```python
from build123d import *

# Parameters (mm, degrees)
F0_W     = 38.1
F0_H     = 38.1
F0_H_2   = 368.3
F0_H_3   = 25.4
F1_DEPTH = 38.1
F2_DEPTH = 800.1
F0_W_2   = 768.35
F3_DEPTH = 38.1


with BuildPart() as f1:
    # F0 (on Top) → F1 (new body)
    with BuildSketch(Plane.XY):
        with Locations((1200.15, 590.55)):
            Rectangle(F0_W, F0_H)
        Polygon((1181.1, 571.5), (1181.1, 609.6), (19.05, 609.6), (19.05, 571.5), (374.65, 571.5), (412.75, 571.5), align=None)
        Polygon((1219.2, -571.5), (1219.2, 571.5), (1181.1, 571.5), (1181.1, 203.2), (1181.1, 177.8), (1181.1, 0), (1181.1, -177.8), (1181.1, -203.2), (1181.1, -571.5), align=None)
        Polygon((19.05, 571.5), (19.05, 609.6), (-19.05, 609.6), (-19.05, 571.5), (0, 571.5), align=None)
        with Locations((1200.15, -590.55)):
            Rectangle(F0_W, F0_H)
        Polygon((-19.05, 571.5), (-19.05, 609.6), (-1181.1, 609.6), (-1181.1, 571.5), (-412.75, 571.5), (-374.65, 571.5), align=None)
        Polygon((1181.1, -609.6), (1181.1, -571.5), (412.75, -571.5), (374.65, -571.5), (19.05, -571.5), (19.05, -609.6), align=None)
        with Locations((-1200.15, 590.55)):
            Rectangle(F0_W, F0_H)
        Polygon((-1181.1, 203.2), (-1181.1, 571.5), (-1219.2, 571.5), (-1219.2, -571.5), (-1181.1, -571.5), (-1181.1, -203.2), (-1181.1, -177.8), (-1181.1, 0), (-1181.1, 177.8), align=None)
        with Locations((0, -590.55)):
            Rectangle(F0_W, F0_H)
        Polygon((-1181.1, -609.6), (-19.05, -609.6), (-19.05, -571.5), (-374.65, -571.5), (-412.75, -571.5), (-1181.1, -571.5), align=None)
        with Locations((-1200.15, -590.55)):
            Rectangle(F0_W, F0_H)
        with Locations((-393.7, 387.35)):
            Rectangle(F0_W, F0_H_2)
        with Locations((-393.7, -387.35)):
            Rectangle(F0_W, F0_H_2)
        with Locations((393.7, 387.35)):
            Rectangle(F0_W, F0_H_2)
        with Locations((393.7, -387.35)):
            Rectangle(F0_W, F0_H_2)
        Polygon((412.75, -177.8), (412.75, 0), (393.7, 0), (374.65, 0), (374.65, -177.8), align=None)
        Polygon((412.75, 0), (412.75, 177.8), (374.65, 177.8), (374.65, 0), (393.7, 0), align=None)
        with Locations((393.7, -190.5)):
            Rectangle(F0_W, F0_H_3)
        with Locations((393.7, 190.5)):
            Rectangle(F0_W, F0_H_3)
        with Locations((-393.7, -190.5)):
            Rectangle(F0_W, F0_H_3)
        Polygon((-374.65, -177.8), (-374.65, 0), (-393.7, 0), (-412.75, 0), (-412.75, -177.8), align=None)
        Polygon((-374.65, 0), (-374.65, 177.8), (-412.75, 177.8), (-412.75, 0), (-393.7, 0), align=None)
        with Locations((-393.7, 190.5)):
            Rectangle(F0_W, F0_H_3)
    extrude(amount=F1_DEPTH)

    # F0 (on Top) → F2 (join)
    with BuildSketch(Plane.XY):
        with Locations((1200.15, 590.55)):
            Rectangle(F0_W, F0_H)
        with Locations((1200.15, -590.55)):
            Rectangle(F0_W, F0_H)
        with Locations((0, -590.55)):
            Rectangle(F0_W, F0_H)
        Polygon((19.05, 571.5), (19.05, 609.6), (-19.05, 609.6), (-19.05, 571.5), (0, 571.5), align=None)
        with Locations((-1200.15, 590.55)):
            Rectangle(F0_W, F0_H)
        with Locations((-1200.15, -590.55)):
            Rectangle(F0_W, F0_H)
    extrude(amount=-F2_DEPTH)

    # F0 (on Top) → F3 (join)
    with BuildSketch(Plane.XY):
        Polygon((-374.65, -203.2), (374.65, -203.2), (374.65, -177.8), (0, -177.8), (-374.65, -177.8), align=None)
        Polygon((374.65, 177.8), (374.65, 203.2), (0, 203.2), (0, 190.5), (0, 177.8), align=None)
        with Locations((-796.925, 190.5)):
            Rectangle(F0_W_2, F0_H_3)
        Polygon((0, 190.5), (0, 203.2), (-374.65, 203.2), (-374.65, 177.8), (0, 177.8), align=None)
        with Locations((-796.925, -190.5)):
            Rectangle(F0_W_2, F0_H_3)
        with Locations((796.925, -190.5)):
            Rectangle(F0_W_2, F0_H_3)
        with Locations((796.925, 190.5)):
            Rectangle(F0_W_2, F0_H_3)
    extrude(amount=F3_DEPTH)


solid = f1.part
```
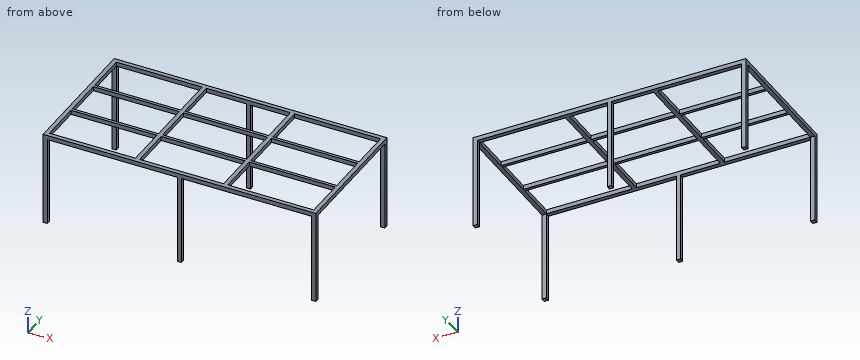
Check sheet for the modelled part. Datum: model origin and axes. Units: mm. Round coordinates to 2 decimals unless told otherwise and drop trailing zeros. Order: outer loops, then holes, each group sorted by start corner. A loop starts at its lowest first (then second) coordinate and runs counter-clockwise, first axis right, second up. Notation, with made-up numbers: (25.5, 19.25) -> (57.5, 19.25) arc R15 cw to (57.5, 30.25) -> close; hole circle Ø9 at (40.25, -9). An arc over 180 degrees is marked (long way). One line per item, written item: value. Start each with the question number.
Q1. Cross-section at A-A (z = -391.5). Record the boundary of the cut face in (x, y), and give its area (3 significant figures).
Q2. Gauge pin test, flat end, axial feed: pin 1 Ø5 at (x, z) = (-22, -183.5) entering from -Y. Record the tip position at first contact, or that the pin passes through.
Q3. Cross-section at B-B (y = -491.5). Record the boundary of the cut face in (x, z).
Q4. Cross-section at C-C (x = -724.5). Record the boundary of the cut face in (y, z), and give its area (3 significant figures).
Completed:
1. outline: (-1219.2, -609.6) -> (-1181.1, -609.6) -> (-1181.1, -571.5) -> (-1219.2, -571.5) -> close; (-1219.2, 571.5) -> (-1181.1, 571.5) -> (-1181.1, 609.6) -> (-1219.2, 609.6) -> close; (-19.05, -609.6) -> (19.05, -609.6) -> (19.05, -571.5) -> (-19.05, -571.5) -> close; (-19.05, 571.5) -> (19.05, 571.5) -> (19.05, 609.6) -> (-19.05, 609.6) -> close; (1181.1, -609.6) -> (1219.2, -609.6) -> (1219.2, -571.5) -> (1181.1, -571.5) -> close; (1181.1, 571.5) -> (1219.2, 571.5) -> (1219.2, 609.6) -> (1181.1, 609.6) -> close
1. area: 8,710 mm²
2. pin 1: passes through
3. outline: (-1219.2, 0) -> (-1181.1, 0) -> (-1181.1, 38.1) -> (-1219.2, 38.1) -> close; (-412.75, 0) -> (-374.65, 0) -> (-374.65, 38.1) -> (-412.75, 38.1) -> close; (374.65, 0) -> (412.75, 0) -> (412.75, 38.1) -> (374.65, 38.1) -> close; (1181.1, 0) -> (1219.2, 0) -> (1219.2, 38.1) -> (1181.1, 38.1) -> close
4. outline: (-609.6, 0) -> (-571.5, 0) -> (-571.5, 38.1) -> (-609.6, 38.1) -> close; (-203.2, 0) -> (-177.8, 0) -> (-177.8, 38.1) -> (-203.2, 38.1) -> close; (177.8, 0) -> (203.2, 0) -> (203.2, 38.1) -> (177.8, 38.1) -> close; (571.5, 0) -> (609.6, 0) -> (609.6, 38.1) -> (571.5, 38.1) -> close
4. area: 4,840 mm²
